Model file for the job. Use its own axes, mm. A direction names the side the tool comes from. Coordinates: 2 decimals unless noted, no trailing zeros. Order: outer loops, then holes, each group sorted by start corner. A loop starts at its lowest first (then second) coordinate and runs counter-clockwise, first axis right, second up. Notation, with made-up numbers: (-18.5, -19) -> (-1.5, -19) arc R18 cw to (-1.5, 14) -> close; hole circle Ø5 at (-24.75, 1.25). An arc over 180 degrees is marked (long way). Write item = value, one per line. Start each with the question number.
Q1. 3-axis set-ups, long thin cutter, end or side, ignore diameter. For faces 1 (the face through (2, 0, 2)), 2 (the face through (140, 35, 120)), 3 (the face through (145, 35, -100)): which of +Z, -Z, +X, -X, +Y, -Y reach the whole face in a straight line?
Q2. Flat gauge pins, fed straight in: pin 1 (15 mm diameter, centred on y = 47, z = -30, fed in from +X); pin 2 (10 mm diameter, centred on x = 37, z = 24, fed in from +Y). Where does each tip first touch, or does it go through?
Q3. Cut at B-B, the plane z = -82.5. List the corners of the cut face in (x, y), plus the area to 3 significant figures.
Q4. Mould opens along Z. For faces 4 (the face through (145, 35, 100)), 5 (the face through (150, 9.6, 35.4)), 6 (the face through (-2, 30, 150)), 7 (the face through (2, 30, -150)) say: +Z half, -Z half, draft (parallel to the pull), parting line (faces both ways), or undercut.
Q5. Cut at D-D, the plane z = 125. List the corners of the cut face in (x, y), plus the area to 3 significant figures.
Q6. Cut at A-A, the plane y = 17. List the corners of the cut face in (x, z), plus the area to 3 significant figures.
Q7. Wall check: line 1 (Z direction, x = -24.5, y = 37.5); line 2 (X direction, y = 42, z = 31.5). Give the ranges that are in metal, low to high. Write a range as from..to.
Q8. Cut at C-C, the plane x = -16. List the corners of the cut face in (y, z).
Autodesk Inventor part; units mm, degrees
ref_plane "YZ Plane" through (0, 0, 0) normal (1, 0, 0) x (0, 1, 0)
ref_plane "XZ Plane" through (0, 0, 0) normal (0, 1, 0) x (-1, 0, 0)
ref_plane "XY Plane" through (0, 0, 0) normal (0, 0, 1) x (1, 0, 0)
sketch "草图1" plane through (0, 0, 0) normal (0, 1, 0) x (-1, 0, 0)
  line L0 (150, 150) -> (-150, 150)
  line L1 (-150, 150) -> (-150, -150)
  line L2 (-150, -150) -> (150, -150)
  line L3 (150, -150) -> (150, 150)
  line L4 (150, 150) -> (-150, -150) construction
  line L5 (-150, 150) -> (150, -150) construction
  point P0 (0, 0)
  dimension "d0" = 300
  dimension "d1" = 300
extrude "拉伸1" add sketch "草图1" along normal blind 10
sketch "草图3" plane through (0, 10, 0) normal (0, 1, 0) x (1, 0, 0)
  line L0 (-150, -150) -> (-150, 150)
  line L1 (-150, 150) -> (150, 150)
  line L2 (150, 150) -> (150, -150)
  line L3 (150, -150) -> (-150, -150)
  line L4 (-140, -140) -> (-140, 140)
  line L5 (-140, 140) -> (140, 140)
  line L6 (140, 140) -> (140, -140)
  line L7 (140, -140) -> (-140, -140)
  point P0 (0, 0)
  dimension "d5" = 10
extrude "拉伸2" add sketch "草图3" along normal blind 50
sketch "草图4" plane through (150, 0, 150) normal (1, 0, 0) x (0, 0, -1)
  line L0 (0, 60) -> (300, 60)
  line L1 (300, 60) -> (300, 0)
  line L2 (300, 0) -> (0, 0)
  line L3 (0, 0) -> (0, 60)
  line L4 (0, 0) -> (0, 60)
  line L5 (0, 60) -> (50, 60)
  line L6 (300, 60) -> (0, 60)
  line L7 (300, 60) -> (250, 60)
  line L8 (50, 60) -> (50, 10)
  line L9 (300, 0) -> (0, 0)
  line L10 (250, 60) -> (250, 10)
  line L11 (290, 10) -> (10, 10)
  line L12 (50, 10) -> (250, 10)
  point P0 (150, 0)
  point P1 (250, 0)
  point P2 (250, 60)
  point P3 (53, 0)
  dimension "d8" = 300
  dimension "d9" = 50
  dimension "d18" = 50
extrude "拉伸3" cut sketch "草图4" against normal blind 10 contours L0 L10 L11 L8
properties part number "放书的" material "聚乙烯，低密度"
Here are the results:
q1.face_1 = +Z, -Z, +X, -X, -Y
q1.face_2 = +Y
q1.face_3 = +X, +Y
q2.pin_1 = -140
q2.pin_2 = 10
q3.outline = (-150, 0) -> (150, 0) -> (150, 10) -> (-140, 10) -> (-140, 60) -> (-150, 60) -> close
q3.area = 3,500 mm²
q4.face_4 = undercut
q4.face_5 = draft
q4.face_6 = +Z half
q4.face_7 = -Z half
q5.outline = (-150, 0) -> (150, 0) -> (150, 60) -> (140, 60) -> (140, 10) -> (-140, 10) -> (-140, 60) -> (-150, 60) -> close
q5.area = 4,000 mm²
q6.outline = (-150, -150) -> (150, -150) -> (150, -100) -> (140, -100) -> (140, -140) -> (-140, -140) -> (-140, 140) -> (140, 140) -> (140, 100) -> (150, 100) -> (150, 150) -> (-150, 150) -> close
q6.area = 9,600 mm²
q7.line_1 = -150..-140, 140..150
q7.line_2 = -150..-140
q8.outline = (0, -150) -> (60, -150) -> (60, -140) -> (10, -140) -> (10, 140) -> (60, 140) -> (60, 150) -> (0, 150) -> close
